Autodesk Inventor part; units mm, degrees
ref_plane "YZ Plane" through (0, 0, 0) normal (1, 0, 0) x (0, 1, 0)
ref_plane "XZ Plane" through (0, 0, 0) normal (0, 1, 0) x (-1, 0, 0)
ref_plane "XY Plane" through (0, 0, 0) normal (0, 0, 1) x (1, 0, 0)
sketch "スケッチ1" plane through (0, 0, 0) normal (0, 0, 1) x (1, 0, 0)
  line L0 (-45, 3.5) -> (45, 3.5)
  line L1 (45, 3.5) -> (45, -3.5)
  line L2 (45, -3.5) -> (-45, -3.5)
  line L3 (-45, -3.5) -> (-45, 3.5)
  line L4 (-45, 3.5) -> (45, -3.5) construction
  line L5 (45, 3.5) -> (-45, -3.5) construction
  point P0 (0, 0)
  dimension "d0" = 90
  dimension "d1" = 7
extrude "押し出し1" add sketch "スケッチ1" along normal blind 3
sketch "スケッチ2" plane through (0, 0, 3) normal (0, 0, 1) x (1, 0, 0)
  circle A0 centre (-41, -0.4) radius 2.9
  circle A1 centre (41, -0.4) radius 2.9
  line L0 (45, 3.5) -> (-45, 3.5)
  line L1 (45, -3.5) -> (45, 3.5)
  point P0 (0, 0)
  dimension "d4" = 5.8
  dimension "d5" = 5.8
  dimension "d7" = 3.9
  dimension "d8" = 3.9
  dimension "d9" = 82
  dimension "d10" = 4
extrude "押し出し2" cut sketch "スケッチ2" against normal blind 2
sketch "スケッチ3" plane through (0, 0, 0) normal (0, 0, -1) x (-1, 0, 0)
  circle A0 centre (41, -0.4) radius 1.5
  circle A1 centre (-41, -0.4) radius 1.5
  line L0 (45, -3.5) -> (45, 3.5)
  line L1 (-45, 3.5) -> (-45, -3.5)
  line L2 (45, 3.5) -> (-45, 3.5)
  point P0 (0, 0)
  dimension "d13" = 3
  dimension "d14" = 3
  dimension "d15" = 4
  dimension "d16" = 4
  dimension "d17" = 3.9
  dimension "d18" = 3.9
extrude "押し出し3" cut sketch "スケッチ3" against normal blind 2
sketch "スケッチ4" plane through (-45, -3.5, 0) normal (0, -1, 0) x (1, 0, 0)
  line L0 (0, 0) -> (90, 0)
  line L1 (90, 0) -> (90, 3)
  line L2 (90, 3) -> (0, 3)
  line L3 (0, 3) -> (0, 0)
  point P0 (45, 0)
extrude "押し出し4" add sketch "スケッチ4" along normal blind 5
fillet "フィレット1" radius 4 1 edges at (0, -8.5, 3)
sketch "スケッチ6" plane through (0, 0, 0) normal (0, 0, -1) x (-1, 0, 0)
  line L0 (37, -0.5) -> (-37, -0.5)
  line L1 (-37, -0.5) -> (-37, 3.5)
  line L2 (-37, 3.5) -> (37, 3.5)
  line L3 (37, 3.5) -> (37, -0.5)
  line L4 (45, -8.5) -> (45, 3.5)
  line L5 (45, 3.5) -> (-45, 3.5)
  point P0 (0, 0)
  dimension "d24" = 74
  dimension "d25" = 8
  dimension "d26" = 0
  dimension "d27" = 4
extrude "押し出し5" cut sketch "スケッチ6" against normal blind 10
properties part number "LineTraceCover"
Here's how the part is built. I have some questions about the finished solid (model axes, mm). A direction names the side the tool comes from. Coordinates: 2 decimals unless noted, no trailing zeros. Order: outer loops, then holes, each group sorted by start corner. A loop starts at its lowest first (then second) coordinate and runs counter-clockwise, first axis right, second up.
1) Imagine slicing it at B-B on z = 2.3. List the corners of the cut face in (x, y) for me, and give its area (3 significant figures).
2) Imagine slicing it at C-C on y = -6.5. List the corners of the cut face in (x, z) for me, and give its area (3 significant figures).
3) Which directions (+Z, -Z, +X, -X, +Y, -Y) give clear straight access to the entire face, cutting with the end or side of a thin tool? Please do faces 4 (the face through (-38.234, 0.471, 2.014)), 5 (the face through (-1, -0.5, 1)), 6 (the face through (45, -2, 1)).
4) Will this pin go through, and if not, where does the flat tip stop? pin 1 (3 mm diameter, centred on x = -41, y = -1.5, fed in from +Z).
5) We'd pull the mould along X, two halves only. Please class faces 1 (the face through (-40, -2, 1)), 2 (the face through (-45, -2, 2)), 3 (the face through (-1, -4, 0)): +X half, -X half, draft (parallel to the pull), parting line (faces both ways), or undercut.
6) Imagine slicing it at A-A on x = -41. List the corners of the cut face in (y, z) for me, and give its area (3 significant figures).
7) I need wall thicknesses on line 1 (X direction, y = -1, z = 2.7); line 2 (Y direction, x = -41, z = 1.7); line 3 (X direction, y = -1, z = 0.6). Which ranges of each line are inside material? Lowest first, please.
Response values:
1. outline: (-45, -6.89) - (45, -6.89) - (45, 3.5) - (37, 3.5) - (37, -0.5) - (-37, -0.5) - (-37, 3.5) - (-45, 3.5) - close; hole circle Ø5.8 at (-41, -0.4); hole circle Ø5.8 at (41, -0.4)
1. area: 586 mm2
2. outline: (-45, 0) - (45, 0) - (45, 2.53) - (-45, 2.53) - close
2. area: 228 mm2
3. face 4: +Z
3. face 5: +Z, -Z, +Y
3. face 6: +Z, -Z, +X, +Y, -Y
4. pin 1: stops at z = 1
5. face 1: undercut
5. face 2: -X half
5. face 3: draft
6. outline: (-8.5, 0) - (-1.9, 0) - (-1.9, 1) - (-3.3, 1) - (-3.3, 3) - (-4.63, 3) arc R4 ccw to start; (1.1, 0) - (3.5, 0) - (3.5, 3) - (2.5, 3) - (2.5, 1) - (1.1, 1) - close
6. area: 18.4 mm2
7. line 1: x = -45 to -43.84, -38.16 to 38.16, 43.84 to 45
7. line 2: y = -7.58 to -3.3, 2.5 to 3.5
7. line 3: x = -45 to -42.37, -39.63 to 39.63, 42.37 to 45
